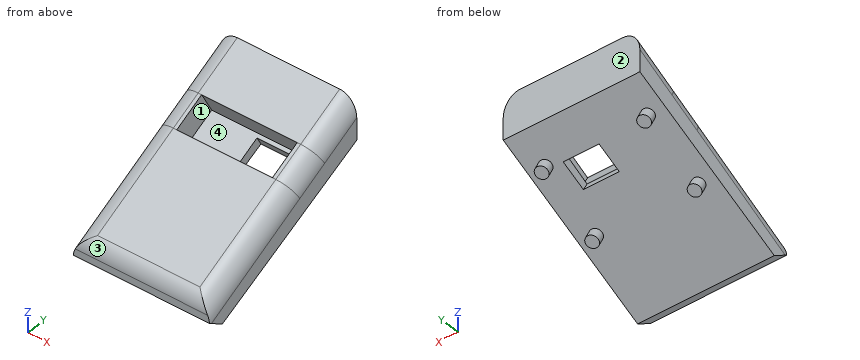
from build123d import *

# Parameters (mm, degrees)
F1_DEPTH = 40
F2_W     = 6
F2_H     = 7.3
F3_DEPTH = 10
F4_W     = 10.5
F4_H     = 8
F5_DEPTH = 25
F6_R     = 1.75
F7_DEPTH = 3
F8_R     = 5
F9_SIZE  = 5


with BuildPart() as f1:
    # F0 (on Right) → F1 (new body)
    with BuildSketch(Plane.YZ):
        Polygon((15.7016541125, 5.8919606872), (15.7016541125, 17.8919606872), (1.959085995, 10.2806947738), (5.4959338209, 3.8947173658), (-3.2519804366, -0.9502796561), (-6.7888282626, 5.435697752), (-36.0735021532, -10.7835007459), (-36.0735021532, -20.7835007459), align=None)
    extrude(amount=F1_DEPTH)

    # F2 (on face) → F3 (join, through all)
    with BuildSketch(Plane(origin=(0, 5.8565406788, 3.2436214293), x_dir=(1, 0, 0), z_dir=(0, -0.8747914258, -0.4844997022))):
        with Locations((3, 4.3942870579)):
            Rectangle(F2_W, F2_H)
        with Locations((37, 4.3942870579)):
            Rectangle(F2_W, F2_H)
    extrude(amount=F3_DEPTH)

    # F4 (on face) → F5 (cut)
    with BuildSketch(Plane(origin=(0, -0.3606068579, 0.6510959365), x_dir=(1, 0, 0), z_dir=(0, -0.4844997022, 0.8747914258))):
        with Locations((25.3092581406, 1.6064377211)):
            Rectangle(F4_W, F4_H)
    extrude(amount=-F5_DEPTH, mode=Mode.SUBTRACT)

    # F6 (on face) → F7 (join)
    with BuildSketch(Plane(origin=(0, 0.8948185727, -1.7367786325), x_dir=(1, 0, 0), z_dir=(0, 0.4580028747, -0.8889507111))):
        with Locations((35, -6.656531521)):
            Circle(F6_R)
        with Locations((5, -6.656531521)):
            Circle(F6_R)
        with Locations((35, 13.343468479)):
            Circle(F6_R)
        with Locations((5, 13.343468479)):
            Circle(F6_R)
    extrude(amount=F7_DEPTH)

    # F8
    f8_edges = [f1.edges().sort_by_distance(p)[0] for p in [
        (20, -36.073502, -10.783501),
        (40, -10.185924, 3.55423),
        (0, -10.185924, 3.55423),
    ]]
    fillet(f8_edges, radius=F8_R)

    # F9
    f9_edges = [f1.edges().sort_by_distance(p)[0] for p in [
        (20, -36.073502, -20.783501),
    ]]
    chamfer(f9_edges, length=F9_SIZE)


solid = f1.part
The listing builds one solid part. Answer for the finished solid, in the listing's coordinates (mm). Face numbers are marked on the shaded views. A direction names the side the tool comes from. Coordinates: 2 decimals unless noted, no trailing zeros. Order: outer loops, then holes, each group sorted by start corner. A loop starts at its lowest first (then second) coordinate and runs counter-clockwise, first axis right, second up. Notation, with made-up numbers: (84, 56) -> (122, 56) arc R13 cw to (122, 64) -> close; hole circle Ø11 at (-20.5, 22.5). An arc over 180 degrees is marked (long way). Answer in a Markdown table with one row per item. Add a question column.
Item 1: Which of the six approach directions +Z, -Z, +X, -X, +Y, -Y give full straight-line access (tool end or side, diameter ignored) to the marked faces 1 and 2?
Item 2: Find the intervals of material crossed by L1, parallel to X at y = -4, z = 4; L2, parallel to Z at x = 29, y = -4.5; L3, parallel to Z at x = 3, y = -4, in increasing order. Write a range as from..to.
Item 3: Find section B-B (x = 11.5). Write down the section's boundary in (y, z), then the cut area to 3 significant figures.
Item 4: Each of these flat-tipped pins is pushed along its axis until it touches: P1, Ø2, axis at y = -8, z = 4, coming from the +X side; P2, Ø1.5, axis at x = 33, z = 11.5, coming from the -Y side; P3, Ø1.5, axis at x = 32, y = 9.5, coming from the -Z side. Where does it stop, or does it pass through?
Item 5: Determine the mould class of the marked faces 3 and 4 for opening direction X: +X half, -X half, draft (parallel to the pull), parting line (faces both ways), or undercut.
Item 6: Find section A-A (x = 25.5). Write down the section's boundary in (y, z).
Result set:
| question | item | result |
|---|---|---|
| 1 | face 1 | none |
| 1 | face 2 | +Z, -Z, +X, -X, +Y |
| 2 | L1 | x = 0.61..6, 34..39.39 |
| 2 | L2 | z = -4.52..1.3 |
| 2 | L3 | z = -4.26..6.5 |
| 3 | outline | (-36.07, -15.78) -> (-31.63, -18.49) -> (15.7, 5.89) -> (15.7, 17.89) -> (1.96, 10.28) -> (5.5, 3.89) -> (-3.25, -0.95) -> (-6.79, 5.44) -> (-33.5, -9.36) arc R5 ccw to (-36.07, -13.73) -> close |
| 3 | area | 484 mm² |
| 4 | P1 | stops at x = 38.73 |
| 4 | P2 | stops at y = 2.81 |
| 4 | P3 | stops at z = 2.31 |
| 5 | face 3 | draft |
| 5 | face 4 | undercut |
| 6 | outline | (-36.07, -15.78) -> (-31.63, -18.49) -> (-1.18, -2.81) -> (-2.45, -0.51) -> (-3.25, -0.95) -> (-6.79, 5.44) -> (-33.5, -9.36) arc R5 ccw to (-36.07, -13.73) -> close; (1.96, 10.28) -> (5.5, 3.89) -> (4.54, 3.37) -> (5.93, 0.86) -> (15.7, 5.89) -> (15.7, 17.89) -> close |
